Job drawing, mm, ordinate dimensions from the low corner. One solid piece. Round coordinates to 2 decimals unless told otherwise and drop trailing zeros. Loops run counter-clockwise (first coordinate to the right, second up) from the corner with the lowest first, then second, coordinate; pieces in that order, holes last. Notation, with made-up numbers: M -32,-26.75 L -26,-26.75 A24 cw -26,7.25 Z; hole C 0.25,37 d7. An arc over 180 degrees is marked long. Use a Markdown table: item, result. Add a question column.
(1) Band-saw the part on B-B, the plane x = 81.5. Write the cut outline in (y, z), and give its area (3 significant figures).
(2) Band-saw the part on A-A, the plane y = 46.5. Write the cut outline in (x, z), and give its area (3 significant figures).
(3) Flat gauge pins, fed straight in: P1, Ø5, axis at x = 7.46, z = 33.92, coming from the -Y side; P2, Ø6, axis at x = 82, y = 102, coming from the -Z side. Where does each tip first touch, or does it go through?
(4) Wall check: L1, parallel to Z at x = 78, y = 112.5. Give the ranges that are in metal, low to high.
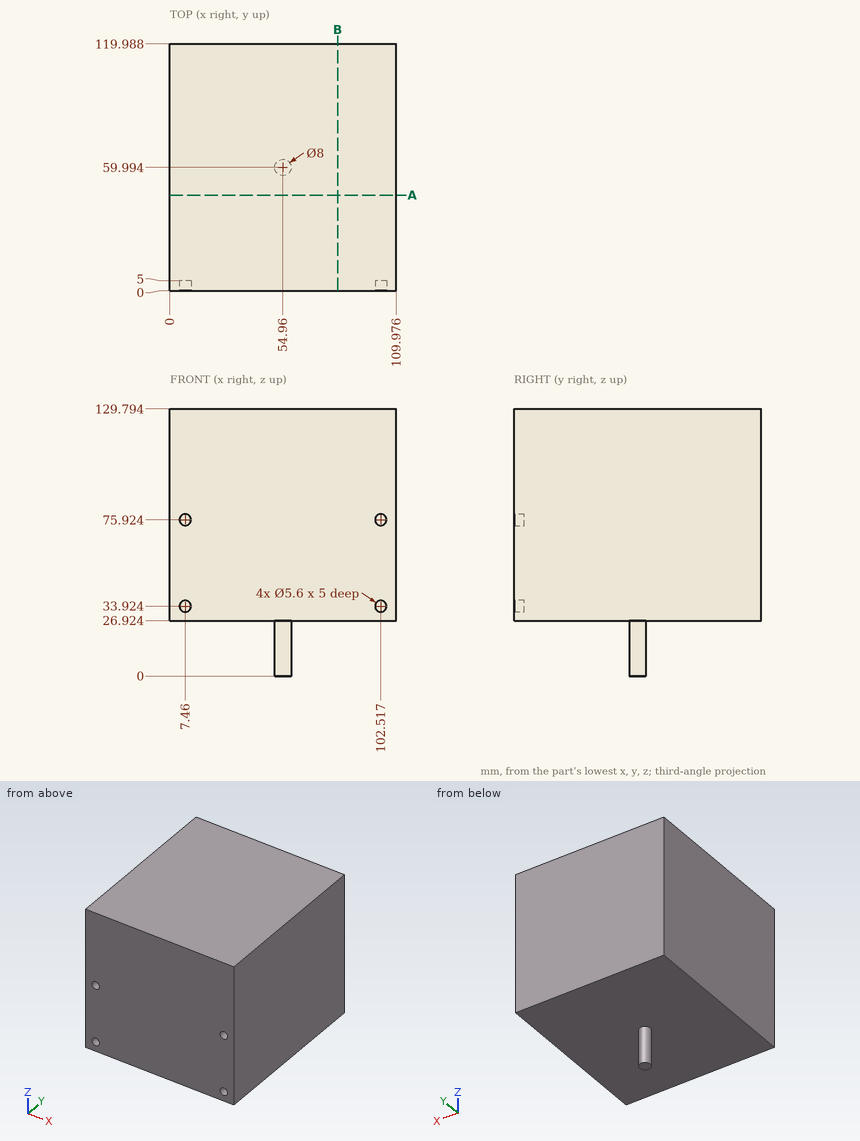
Return value:
| question | item | result |
|---|---|---|
| 1 | outline | M 0,26.92 L 119.99,26.92 L 119.99,129.79 L 0,129.79 Z |
| 1 | area | 12,300 mm^2 |
| 2 | outline | M 0,26.92 L 109.98,26.92 L 109.98,129.79 L 0,129.79 Z |
| 2 | area | 11,300 mm^2 |
| 3 | P1 | y = 5 |
| 3 | P2 | z = 26.92 |
| 4 | L1 | 26.92 to 129.79 |
